Build history of the part. All positions in model axes, mm. A direction names the side the tool comes from. Give positions to 0.01 mm unless a question says otherwise; leave off trailing zeros. Write each loop counter-clockwise with the first axis right and the second up, starting at its lowest first coordinate (ties: lowest second). Pieces come first, ordered by that corner, then holes. Notation, with made-up numbers: (65.5, 34.25) -> (115.5, 34.25) arc R17 cw to (115.5, 49.25) -> close; hole circle Ø1 at (-19, 5). An arc over 180 degrees is marked (long way). One line per question, with ' | ' between items. Start each with the question number.
(1) Band-saw the part on A-A, the plane y = 0. Give the cut face in (x, z) (3 decimals).
(2) Tool access for faces 5 (the flat face through (1, -3, 4.5)), 6 (the flat face through (4.3, -2.1, 2.5)): list every direction of +Z, -Z, +X, -X, +Y, -Y with a clear straight run to the whole face (end or side of a thin tool).
(3) Band-saw the part on C-C, the plane y = 7. Give the cut face in (x, z), and give its area (3 significant figures).
(4) Pull direction X, two halves, no side cores. Call faces 1 (the cylindrical face through (-0.325, -8.464, 1.232)), 2 (the cylindrical face through (5.5, 0.07, 1.23)), 3 (the flat face through (-2.4, -2.1, 0)), 4 (the cylindrical face through (9.514, 2.996, 1.232)): released by +X, released by -X, zero draft, split by the parting line, or undercut.
(5) Pin check, flat tips, straight feed: P1, Ø1.5, axis at y = -7.5, z = 2, coming from the +X side; P2, Ø2, axis at x = 2, z = 2, coming from the +Y side; P3, Ø2, axis at x = -8, z = 2.5, coming from the -Y side. Stop position of each tip, or through.
(6) Drill centre lines: probe 1 along Y at (x, z) = (0, 1.7) (3 decimals); probe 2 along Z at (x, y) = (3, -4); probe 3 along X at (y, z) = (2.75, 2.9). Where is each one in solid material? Low to high. Write a range as from..to.
(7) Band-saw the part on D-D, the plane z = 3.1. Give the cut face in (x, y).
from build123d import *

# Parameters (mm, degrees)
SKETCH1_R           = 9.975
SKETCH1_R_2         = 1.5
BOSS_EXTRUDE1_DEPTH = 2.5
SKETCH2_R           = 4.5
BOSS_EXTRUDE2_DEPTH = 2
SKETCH3_R           = 3
CUT_EXTRUDE1_DEPTH  = 15.807135104


with BuildPart() as part:
    # Sketch1 → Boss-Extrude1 (new body)
    with BuildSketch(Plane.XY):
        Circle(SKETCH1_R)
        with Locations((0, 7)):
            Circle(SKETCH1_R_2, mode=Mode.SUBTRACT)
        with Locations((7, 0)):
            Circle(SKETCH1_R_2, mode=Mode.SUBTRACT)
        with Locations((0, -7)):
            Circle(SKETCH1_R_2, mode=Mode.SUBTRACT)
        with Locations((-7, 0)):
            Circle(SKETCH1_R_2, mode=Mode.SUBTRACT)
    extrude(amount=BOSS_EXTRUDE1_DEPTH)

    # Sketch2 → Boss-Extrude2 (add)
    with BuildSketch(Plane.XY.offset(2.5)):
        Circle(SKETCH2_R)
    extrude(amount=BOSS_EXTRUDE2_DEPTH)

    # Sketch3 → Cut-Extrude1 (cut, through all)
    with BuildSketch(Plane.XY.offset(4.5)):
        Circle(SKETCH3_R)
    extrude(amount=-CUT_EXTRUDE1_DEPTH, mode=Mode.SUBTRACT)


solid = part.part
Results:
1) outline: (-9.975, 0) -> (-8.5, 0) -> (-8.5, 2.5) -> (-9.975, 2.5) -> close; (-5.5, 0) -> (-3, 0) -> (-3, 4.5) -> (-4.5, 4.5) -> (-4.5, 2.5) -> (-5.5, 2.5) -> close; (3, 0) -> (5.5, 0) -> (5.5, 2.5) -> (4.5, 2.5) -> (4.5, 4.5) -> (3, 4.5) -> close; (8.5, 0) -> (9.975, 0) -> (9.975, 2.5) -> (8.5, 2.5) -> close
2) face 5: +Z, +X, -X, +Y, -Y | face 6: +Z
3) outline: (-7.11, 0) -> (-1.5, 0) -> (-1.5, 2.5) -> (-7.11, 2.5) -> close; (1.5, 0) -> (7.11, 0) -> (7.11, 2.5) -> (1.5, 2.5) -> close | area: 28.0 mm²
4) face 1: undercut | face 2: undercut | face 3: zero draft | face 4: split by the parting line
5) P1: stops at x = 7.34 | P2: stops at y = 9.92 | P3: stops at y = -7.11
6) probe 1: y = -9.975..-8.5, -5.5..-3, 3..5.5, 8.5..9.975 | probe 2: z = 0..2.5 | probe 3: x = -3.56..-1.2, 1.2..3.56
7) outline: circle Ø9 at (0, 0); hole circle Ø6 at (0, 0)
